For this review, take the finished solid that the model builds, in its own axes (mm). Face numbers are marked on the shaded views. A direction names the side the tool comes from. Coordinates: 2 decimals unless noted, no trailing zeros. Loops run counter-clockwise (first coordinate to the right, second up) from the corner with the lowest first, then second, coordinate; pieces in that order, holes last. Notation, with made-up numbers: M 61.5,38.25 L 97.5,38.25 A14 cw 97.5,62.25 Z; hole C -26,-35 d4. An arc over 180 degrees is marked long. Write item = value, one per line.
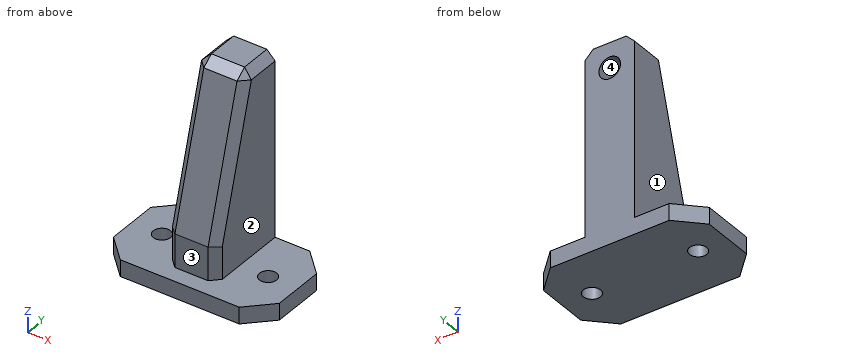
from build123d import *

# Parameters (mm, degrees)
PAD_DEPTH       = 5
PAD001_DEPTH    = 7.5
CHAMFER_SIZE    = 2.5
SKETCH002_R     = 3.25
POCKET_DEPTH    = 11
SKETCH003_R     = 2.6
POCKET001_DEPTH = 5


with BuildPart() as part:
    # Sketch → Pad (new body)
    with BuildSketch(Plane.XY):
        Polygon((-17.928932, -15), (17.928932, -15), (25, -7.928932), (25, 7.928932), (17.928932, 15), (-17.928932, 15), (-25, 7.928932), (-25, -7.928932), align=None)
    extrude(amount=PAD_DEPTH)

    # Sketch001 → Pad001 (join, symmetric)
    with BuildSketch(Plane.YZ):
        Polygon((0, 0), (-10, 0), (-10, 15), (3, 60), (15, 60), (15, 0), align=None)
    extrude(amount=PAD001_DEPTH, both=True)

    # Chamfer
    chamfer_edges = [part.edges().sort_by_distance(p)[0] for p in [
        (0, 3, 60),
        (7.5, -3.5, 37.5),
        (-7.5, -3.5, 37.5),
        (-7.5, -10, 10),
        (7.5, -10, 10),
        (7.5, 9, 60),
        (-7.5, 9, 60),
    ]]
    chamfer(chamfer_edges, length=CHAMFER_SIZE)

    # Sketch002 (on Face4 of Chamfer) → Pocket (cut)
    with BuildSketch(Plane(origin=(0, 15, 0), x_dir=(-1, 0, 0), z_dir=(0, 1, 0))):
        with Locations((0, 52.5)):
            Circle(SKETCH002_R)
    extrude(amount=-POCKET_DEPTH, mode=Mode.SUBTRACT)

    # Sketch003 (on Face19 of Pocket) → Pocket001 (cut)
    with BuildSketch(Plane(origin=(0, 0, 0), x_dir=(1, 0, 0), z_dir=(0, 0, -1))):
        with Locations((-16, 0)):
            Circle(SKETCH003_R)
        with Locations((16, 0)):
            Circle(SKETCH003_R)
    extrude(amount=-POCKET001_DEPTH, mode=Mode.SUBTRACT)


solid = part.part
Q1. Machinability: for the marked faces 1, 2, 3 and 4, which of the approach directions +Z, -Z, +X, -X, +Y, -Y give a long, thin tool a straight path to every point of the face, cutting with its end or side? Answer none if there is none.
Solved:
face_1 = +Z, -X, +Y, -Y
face_2 = +Z, +X, +Y, -Y
face_3 = +Z, +X, -X, -Y
face_4 = +Y
Q2. For pin 1 Ø1.5 at (x, y) = (19, 12) entering from +Z; pin 2 Ø3 at (y, z) = (9.5, 23) entering from +X; pin 3 Ø4 at (y, z) = (1.5, 30.5) entering from -X, all flat-tipped, find the tip position at first contact; note any pin that passes through.
Solved:
pin_1 = 5
pin_2 = 7.5
pin_3 = -7.5
Q3. Add section A-A (x = -16). Write out the cut boundary in (y, z).
Solved:
outline = M -15,0 L -2.6,0 L -2.6,5 L -15,5 Z; M 2.6,0 L 15,0 L 15,5 L 2.6,5 Z
Q4. Add section C-C (x = 0). Write out the cut boundary in (y, z), and give its area (3 significant figures).
Solved:
outline = M -15,0 L 15,0 L 15,49.25 L 4,49.25 L 4,55.75 L 15,55.75 L 15,60 L 5.5,60 L 2.31,57.6 L -10,15 L -10,5 L -15,5 Z
area = 1,160 mm²
Q5. For line 1 along Y through (x, z) = (-16, 3.4); line 2 along Z through (x, y) = (0, 11.75); line 3 along Y through (x, z) = (5, 6.5), list the stretches that pass through material, from the lowest coordinate up.
Solved:
line_1 = -15 to -2.6, 2.6 to 15
line_2 = 0 to 49.25, 55.75 to 60
line_3 = -10 to 15
Q6. Add section D-D (z = 11). Write out the cut boundary in (x, y), and give its area (3 significant figures).
Solved:
outline = M -7.5,-7.5 L -5,-10 L 5,-10 L 7.5,-7.5 L 7.5,15 L -7.5,15 Z
area = 369 mm²
Q7. Add section B-B (y = -1.25). Write out the cut boundary in (x, z).
Solved:
outline = M -25,0 L -18.28,0 L -18.28,5 L -25,5 Z; M -13.72,0 L 13.72,0 L 13.72,5 L 7.5,5 L 7.5,36.28 L 5,45.29 L -5,45.29 L -7.5,36.28 L -7.5,5 L -13.72,5 Z; M 18.28,0 L 25,0 L 25,5 L 18.28,5 Z
